Check sheet for the drawn part. Datum: minimum x, y, z corner. Units: mm. A direction names the side the tool comes from. Coordinates: 2 decimals unless noted, no trailing zeros. Write each loop counter-clockwise with the first axis right and the second up, starting at its lowest first coordinate (ties: lowest second). Pieces come first, ordered by that corner, then holes. Notation, with made-up numbers: (31.5, 58.5) -> (48.5, 58.5) arc R21 ccw to (48.5, 79.5) -> close; hole circle Ø9 at (31.5, -33). An arc over 180 degrees is marked (long way). One line per question, with ' | ' between items.
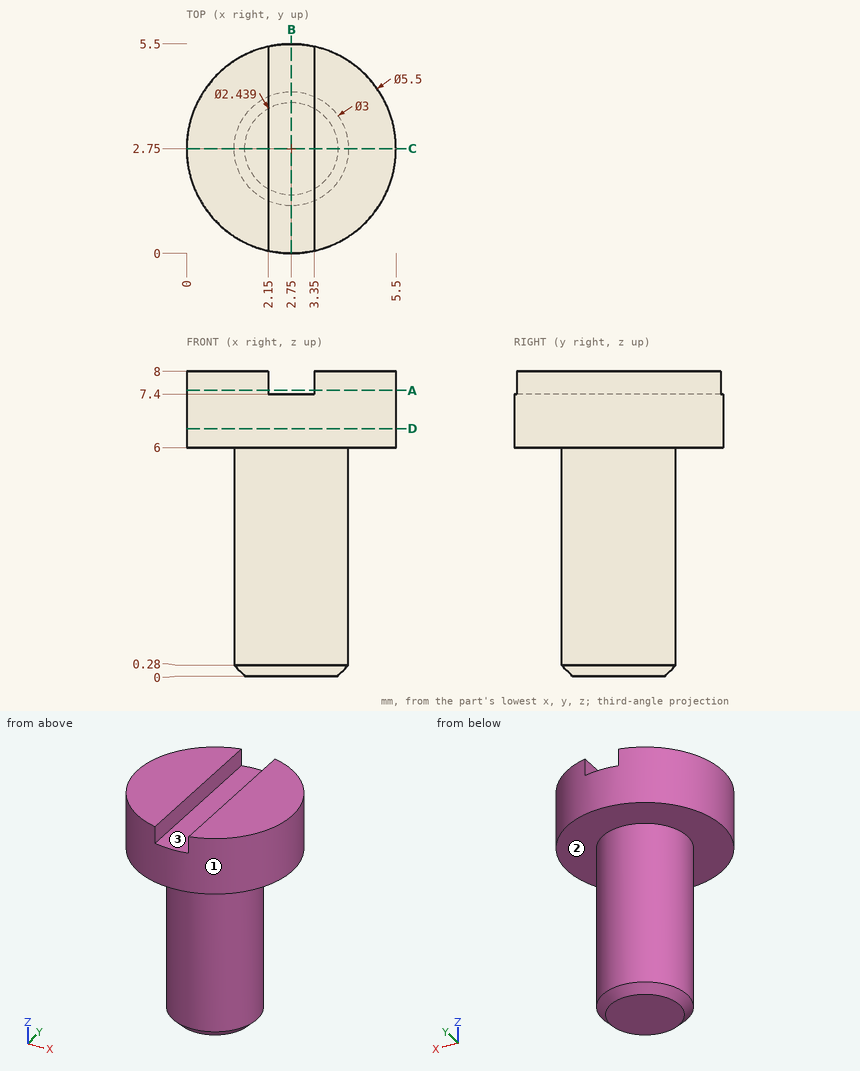
1. Cross-section at D-D on z = 6.5. Record the boundary of the cut face in (x, y).
Worked answers:
outline: circle Ø5.5 at (2.75, 2.75)
2. Material ranges on line 1 (Z direction, x = 0.55, y = 3.1); line 2 (X direction, y = 2.8, z = 1.75); line 3 (Z direction, x = 3.25, y = 1.8), recorded low to high. Write a range as from..to.
Worked answers:
line 1: 6..8 | line 2: 1.25..4.25 | line 3: 0..7.4
3. Go/stop test with a flat-tipped pin: P1, Ø2, axis at y = 1, z = 7, coming from the +X side (1 decimal). Record where the tip stops, or that it passes through.
Worked answers:
P1: x = 5.4
4. Cross-section at C-C on y = 2.75. Record the boundary of the cut face in (x, z), and give its area (3 significant figures).
Worked answers:
outline: (0, 6) -> (1.25, 6) -> (1.25, 0.28) -> (1.53, 0) -> (3.97, 0) -> (4.25, 0.28) -> (4.25, 6) -> (5.5, 6) -> (5.5, 8) -> (3.35, 8) -> (3.35, 7.4) -> (2.15, 7.4) -> (2.15, 8) -> (0, 8) -> close | area: 28.2 mm²
5. Cross-section at A-A on z = 7.5. Record the boundary of the cut face in (x, y), and give its area (3 significant figures).
Worked answers:
outline: (2.15, 0.07) -> (2.15, 5.43) arc R2.75 ccw to start; (3.35, 0.07) arc R2.75 ccw to (3.35, 5.43) -> close | area: 17.2 mm²
6. Tool access check on the marked faces 1, 2 and 3. Record the directions out of +Z, -Z, +X, -X, +Y, -Y that give a thin tool (end or side, any length) a straight path to the whole face; none if there is none.
Worked answers:
face 1: +Z, -Z | face 2: -Z | face 3: +Z, +Y, -Y
7. Cross-section at B-B on x = 2.75. Record the boundary of the cut face in (y, z), and give its area (3 significant figures).
Worked answers:
outline: (0, 6) -> (1.25, 6) -> (1.25, 0.28) -> (1.53, 0) -> (3.97, 0) -> (4.25, 0.28) -> (4.25, 6) -> (5.5, 6) -> (5.5, 7.4) -> (0, 7.4) -> close | area: 25.6 mm²
